```python
from build123d import *

# Parameters (mm, degrees)
SKETCH1_W           = 250
SKETCH1_H           = 66
SKETCH1_R           = 2.5
BOSS_EXTRUDE1_DEPTH = 15


with BuildPart() as part:
    # Sketch1 → Boss-Extrude1 (new body)
    with BuildSketch(Plane.XY):
        with Locations((-22.5, -38.75)):
            Rectangle(SKETCH1_W, SKETCH1_H)
        with Locations((14.728679071, -20)):
            Circle(SKETCH1_R, mode=Mode.SUBTRACT)
        with Locations((14.728679071, -57.5)):
            Circle(SKETCH1_R, mode=Mode.SUBTRACT)
        with Locations((-14.728679071, -57.5)):
            Circle(SKETCH1_R, mode=Mode.SUBTRACT)
        with Locations((-14.728679071, -20)):
            Circle(SKETCH1_R, mode=Mode.SUBTRACT)
        with Locations((-30.271320929, -20)):
            Circle(SKETCH1_R, mode=Mode.SUBTRACT)
        with Locations((-30.271320929, -57.5)):
            Circle(SKETCH1_R, mode=Mode.SUBTRACT)
        with Locations((-59.728679071, -57.5)):
            Circle(SKETCH1_R, mode=Mode.SUBTRACT)
        with Locations((-59.728679071, -20)):
            Circle(SKETCH1_R, mode=Mode.SUBTRACT)
        with Locations((80, -38.75)):
            Circle(SKETCH1_R, mode=Mode.SUBTRACT)
        with Locations(Location((-125, -38.75, 0), (0, 0, 180))):
            Circle(SKETCH1_R, mode=Mode.SUBTRACT)
    extrude(amount=BOSS_EXTRUDE1_DEPTH)


solid = part.part
```
Work out the finished part from the listing and answer in its coordinate system (mm). Give positions to 0.01 mm unless a question says otherwise; leave off trailing zeros. Loops run counter-clockwise (first coordinate to the right, second up) from the corner with the lowest first, then second, coordinate; pieces in that order, holes last. Notation, with made-up numbers: (84, -34.75) -> (115, -34.75) arc R12 ccw to (115, -24.75) -> close; hole circle Ø6 at (23.25, -24). An arc over 180 degrees is marked (long way). Put each result on its own line as item: value. Start each with the question number.
Item 1: The mould has two halves that part along Y. Classify faces 1 (the face through (-24, -71.75, 7)), 2 (the face through (102.5, -39, 7)), 3 (the face through (16.07, -55.39, 7.4)): released by +Y, released by -Y, zero draft, split by the parting line, or undercut.
Item 2: Find the intervals of material crossed by L1, parallel to X at y = -58, z = 5; L2, parallel to X at y = -18, z = 8.5; L3, parallel to Y at x = -60.5, z = 4.75, in increasing order. Write a range as [from, to].
Item 3: This flat-tipped pin is pushed along its axis until it touches: P1, Ø3, axis at x = -30.27, y = -20, coming from the +Z side. Where does it stop, or does it pass through?
Item 4: The part is cut by section B-B (y = -57.5). Give the vertices of the cut face in (x, z).
Item 5: The part is cut by section A-A (y = -38.75). Give the vertices of the cut face in (x, z).
Item 6: The part is cut by section C-C (x = 80). Give the vertices of the cut face in (y, z), then the cut area to 3 significant figures.
Answers below:
1. face 1: released by -Y
1. face 2: zero draft
1. face 3: undercut
2. L1: [-147.5, -62.18], [-57.28, -32.72], [-27.82, -17.18], [-12.28, 12.28], [17.18, 102.5]
2. L2: [-147.5, -61.23], [-58.23, -31.77], [-28.77, -16.23], [-13.23, 13.23], [16.23, 102.5]
2. L3: [-71.75, -59.88], [-55.12, -22.38], [-17.62, -5.75]
3. P1: through
4. outline: (-147.5, 0) -> (-62.23, 0) -> (-62.23, 15) -> (-147.5, 15) -> close; (-57.23, 0) -> (-32.77, 0) -> (-32.77, 15) -> (-57.23, 15) -> close; (-27.77, 0) -> (-17.23, 0) -> (-17.23, 15) -> (-27.77, 15) -> close; (-12.23, 0) -> (12.23, 0) -> (12.23, 15) -> (-12.23, 15) -> close; (17.23, 0) -> (102.5, 0) -> (102.5, 15) -> (17.23, 15) -> close
5. outline: (-147.5, 0) -> (-127.5, 0) -> (-127.5, 15) -> (-147.5, 15) -> close; (-122.5, 0) -> (77.5, 0) -> (77.5, 15) -> (-122.5, 15) -> close; (82.5, 0) -> (102.5, 0) -> (102.5, 15) -> (82.5, 15) -> close
6. outline: (-71.75, 0) -> (-41.25, 0) -> (-41.25, 15) -> (-71.75, 15) -> close; (-36.25, 0) -> (-5.75, 0) -> (-5.75, 15) -> (-36.25, 15) -> close
6. area: 915 mm2
